from build123d import *

# Parameters (mm, degrees)
LINEAR_AUSTRAGEN_D_NN1_DEPTH         = 0.6
LINEAR_AUSTRAGEN_D_NN2_DEPTH         = 14
LINEAR_AUSTRAGEN_D_NN2_DRAFT         = -9
SCHNITT_LINEAR_AUSTRAGEN_D_NN1_DEPTH = 16
SCHNITT_LINEAR_AUSTRAGEN_D_NN1_DRAFT = 9


with BuildPart() as part:
    # Skizze1 → Linear-Austragen-Dünn1 (new body)
    with BuildSketch(Plane.XY):
        Polygon((19.865941325, 0), (11.758199437, 5.817213911), (-12.503529969, 5.817213911), (-19.865941325, 0), (-11.77637823, -5.817213911), (-11.17637823, -5.817213911), (-3.47637823, -5.817213911), (4.22362177, -5.817213911), (11.92362177, -5.817213911), (12.503529969, -5.817213911), align=None)
        Polygon((18.204210014, -0.038494533), (11.436566371, 4.817213911), (-12.156143301, 4.817213911), (-18.205362025, 0.037584302), (-11.45415826, -4.817213911), (-11.17637823, -4.817213911), (-3.47637823, -4.817213911), (4.22362177, -4.817213911), (11.92362177, -4.817213911), (12.156143301, -4.817213911), align=None, mode=Mode.SUBTRACT)
    extrude(amount=LINEAR_AUSTRAGEN_D_NN1_DEPTH)


with BuildPart() as linear_austragen_d_nn2_tool:
    # Skizze2 → Linear-Austragen-Dünn2 (with draft: the straight prism first)
    with BuildSketch(Plane.XY.offset(0.6)):
        Polygon((-12.503529969, 5.817213911), (-19.865941325, 0), (-11.77637823, -5.817213911), (12.503529969, -5.817213911), (19.865941325, 0), (11.758199437, 5.817213911), align=None)
        Polygon((-12.156143301, 4.817213911), (-18.205362025, 0.037584302), (-11.45415826, -4.817213911), (12.156143301, -4.817213911), (18.204210014, -0.038494533), (11.436566371, 4.817213911), align=None, mode=Mode.SUBTRACT)
    extrude(amount=LINEAR_AUSTRAGEN_D_NN2_DEPTH)
    # Linear-Austragen-Dünn2: the draft: its side faces are tilted about the plane it starts from
    linear_austragen_d_nn2_sides = [linear_austragen_d_nn2_tool.faces().sort_by_distance(p)[0] for p in [
        (-16.184735647, 2.908606956, 7.6),
        (-15.821159778, -2.908606956, 7.6),
        (0.363575869, -5.817213911, 7.6),
        (16.184735647, -2.908606956, 7.6),
        (15.812070381, 2.908606956, 7.6),
        (-0.372665266, 5.817213911, 7.6),
        (-0.359788465, 4.817213911, 7.6),
        (14.820388192, 2.389359689, 7.6),
        (15.180176658, -2.427854222, 7.6),
        (0.35099252, -4.817213911, 7.6),
        (-14.829760143, -2.389814805, 7.6),
        (-15.180752663, 2.427399106, 7.6),
    ]]
    draft(linear_austragen_d_nn2_sides, Plane.XY.offset(0.6), LINEAR_AUSTRAGEN_D_NN2_DRAFT)


with BuildPart() as part_1:
    add(part.part)

    # Linear-Austragen-Dünn2: add linear_austragen_d_nn2_tool
    add(linear_austragen_d_nn2_tool.part)


with BuildPart() as schnitt_linear_austragen_d_nn1_tool:
    # Skizze3 → Schnitt-Linear-Austragen-Dünn1 (with draft: the straight prism first)
    with BuildSketch(Plane(origin=(0, 0, 0), x_dir=(-1, 0, 0), z_dir=(0, 0, -1))):
        Polygon((-20.862980112, 0.02309672), (-12.71196197, -6.417213911), (11.969710212, -6.417213911), (20.862288905, -0.022550581), (12.71196197, 6.417213911), (-11.951179276, 6.417213911), align=None)
        Polygon((-19.865941325, 0), (-12.503529969, -5.817213911), (11.77637823, -5.817213911), (19.865941325, 0), (12.503529969, 5.817213911), (-11.758199437, 5.817213911), align=None, mode=Mode.SUBTRACT)
    extrude(amount=-SCHNITT_LINEAR_AUSTRAGEN_D_NN1_DEPTH)
    # Schnitt-Linear-Austragen-Dünn1: the draft: its side faces are tilted about the plane it starts from
    schnitt_linear_austragen_d_nn1_sides = [schnitt_linear_austragen_d_nn1_tool.faces().sort_by_distance(p)[0] for p in [
        (16.787471041, -3.197058596, 8),
        (0.371125879, -6.417213911, 8),
        (-16.415999558, -3.219882246, 8),
        (-16.787125437, 3.197331665, 8),
        (-0.380391347, 6.417213911, 8),
        (16.407079694, 3.220155315, 8),
        (15.812070381, 2.908606956, 8),
        (-0.372665266, 5.817213911, 8),
        (-16.184735647, 2.908606956, 8),
        (-15.821159778, -2.908606956, 8),
        (0.363575869, -5.817213911, 8),
        (16.184735647, -2.908606956, 8),
    ]]
    draft(schnitt_linear_austragen_d_nn1_sides, Plane(origin=(0, 0, 0), x_dir=(-1, 0, 0), z_dir=(0, 0, -1)), SCHNITT_LINEAR_AUSTRAGEN_D_NN1_DRAFT)


with BuildPart() as part_2:
    add(part_1.part)

    # Schnitt-Linear-Austragen-Dünn1: cut by schnitt_linear_austragen_d_nn1_tool
    add(schnitt_linear_austragen_d_nn1_tool.part, mode=Mode.SUBTRACT)


solid = part_2.part
Can you work these out from the model? Positions are in its coordinate system, mm. A direction names the side the tool comes from. Coordinates: 2 decimals unless noted, no trailing zeros. Write each loop counter-clockwise with the first axis right and the second up, starting at its lowest first coordinate (ties: lowest second). Pieces come first, ordered by that corner, then holes. Notation, with made-up numbers: (67.25, 18.25) -> (110.25, 18.25) arc R14 cw to (110.25, 25.25) -> close; hole circle Ø3 at (52.5, 51). An arc over 180 degrees is marked (long way). Write each question's results on one line, items separated by ' | '. Start each with the question number.
Item 1: If we section it at C-C, the plane z = 2.5: Write out the boundary of the cut face in (x, y).
Item 2: I'm going to push flat-ended pins straight in: P1, Ø2, axis at x = 0, z = 9, coming from the -Y side; P2, Ø4, axis at x = -1.5, z = 9, coming from the -Y side; P3, Ø1, axis at x = -15.5, z = 3, coming from the +Y side. Where does each tip first touch, or does it pass through?
Item 3: If we section it at D-D, the plane y = 3: Write out the boundary of the cut face in (x, z), and give its area (3 significant figures).
Item 4: If we section it at B-B, the plane y = 0.5: Write out the boundary of the cut face in (x, z).
Item 5: If we section it at A-A, the plane x = -5: Write out the boundary of the cut face in (y, z), and give its area (3 significant figures).
Item 6: Please list where these lines run through material, in increasing order: probe 1 along Y at (x, z) = (16, 7.5); probe 2 along X at (y, z) = (4, 2); probe 3 along Y at (x, z) = (14, 11.75).
Item 7: On a 3-axis mill with a long thin cutter (end or side, diameter ignored), from which of +Z, -Z, +X, -X, +Y, -Y can I reach the whole of each face in a straight line? I mean faces 5 (the flat face through (-15.099, -2.024, 7.198)), 6 (the flat face through (-14.61, 1.8, 5.95)). Say none if no direction works.
Item 8: Thinking about a two-plate mould opening in Y: for faces 1 (the flat face through (-0.195, 3.724, 7.502)), 2 (the flat face through (15.091, 2.023, 7.198)), 3 (the flat face through (14.71, -2.62, 7.2)), 4 (the flat face through (13.479, 2.007, 7.502)), which applies, released by +Y, released by -Y, zero draft, split by the parting line, or undercut?
Answer block:
1) outline: (-19.21, 0.01) -> (-11.65, -5.42) -> (12.37, -5.42) -> (19.21, -0.02) -> (11.63, 5.42) -> (-12.37, 5.42) -> close; hole (-17.71, 0.05) -> (-11.36, -4.52) -> (12.05, -4.52) -> (17.7, -0.05) -> (11.34, 4.52) -> (-12.05, 4.52) -> close
2) P1: y = -4.55 | P2: y = -4.71 | P3: y = 3.25
3) outline: (-16.07, 0) -> (-14.46, 0) -> (-14.46, 0.6) -> (-11.52, 12.07) -> (10.85, 12.07) -> (13.97, 0.6) -> (13.97, 0) -> (15.68, 0) -> (11.72, 14.6) -> (-12.34, 14.6) -> close | area: 98.9 mm²
4) outline: (-19.23, 0) -> (-17.62, 0) -> (-17.62, 0.6) -> (-14.04, 14.6) -> (-15.5, 14.6) -> close; (13.65, 14.6) -> (17.45, 0.6) -> (17.45, 0) -> (19.17, 0) -> (15.2, 14.6) -> close
5) outline: (-5.82, 0) -> (-4.82, 0) -> (-4.82, 0.6) -> (-2.6, 14.6) -> (-3.5, 14.6) -> close; (2.6, 14.6) -> (4.82, 0.6) -> (4.82, 0) -> (5.82, 0) -> (3.5, 14.6) -> close | area: 26.5 mm²
6) probe 1: -1.54 to -0.39, 0.2 to 1.31 | probe 2: -14.29 to -12.83, 12.2 to 13.75 | probe 3: -2.26 to -1.11, 0.8 to 1.92
7) face 5: +Z, -X, -Y | face 6: -Z
8) face 1: undercut | face 2: released by +Y | face 3: released by -Y | face 4: undercut
